Design review of the part shown in the three views and the two pictorial views. Dimensions are in mm from the part's minimum x, y and z. A direction names the side the tool comes from. Give positions to 0.01 mm unless a question says otherwise; leave off trailing zeros. Write each loop counter-clockwise with the first axis right and the second up, starting at its lowest first coordinate (ties: lowest second). Pieces come first, ordered by that corner, then holes. Notation, with made-up numbers: (80, 5.25) -> (94, 5.25) arc R18 cw to (94, 25.25) -> close; hole circle Ø5 at (10.5, 86.25). An arc over 180 degrees is marked (long way). Return JSON: item names as keys, results as strings. Group by question number.
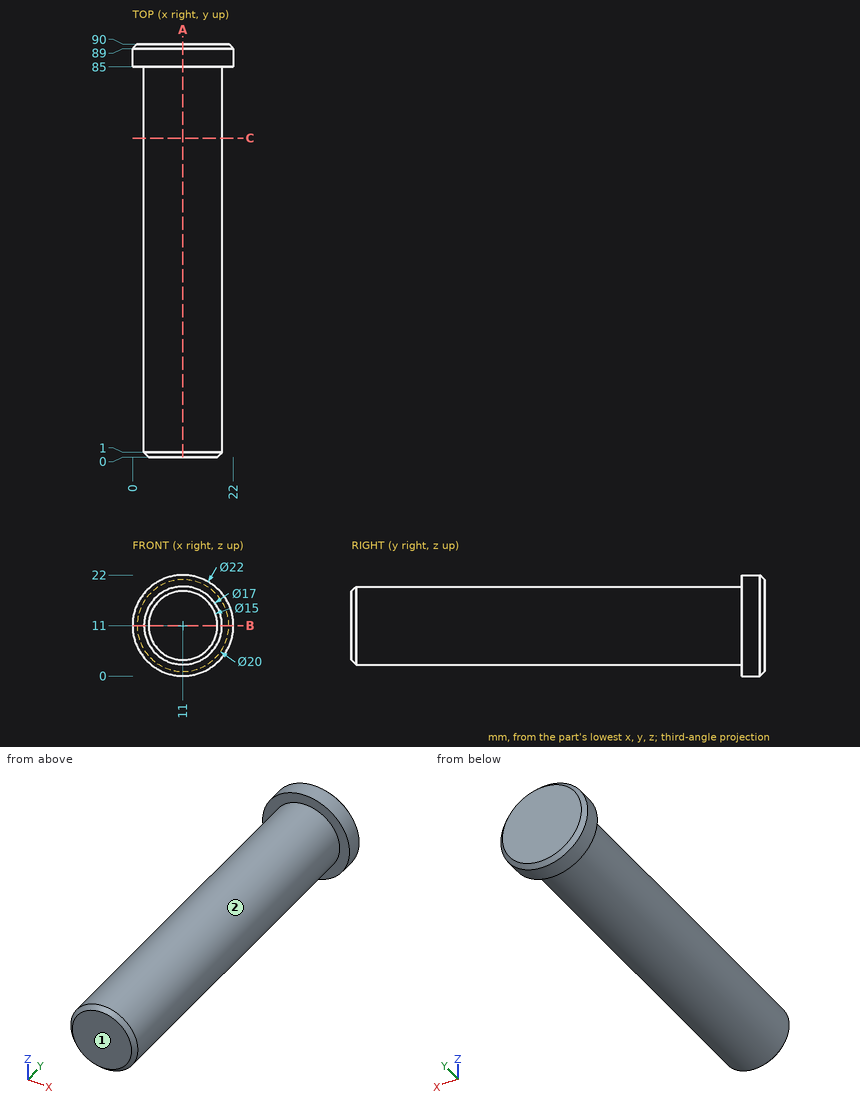
Q1. Take a section at C-C, the plane y = 69.5. Give the boundary of the cut face in (x, z).
Q2. Take a section at A-A, the plane x = 11. Give the boundary of the cut face in (y, z), plus the area to 3 significant figures.
Q3. Tool access review of the marked faces 1 and 2: name each direction out of +Z, -Z, +X, -X, +Y, -Y from which nothing blocks a thin tool from reaching the whole face with its end or side.
Q4. Take a section at B-B, the plane z = 11. Give the boundary of the cut face in (x, y), plus the area to 3 significant figures.
Q5. For L1, parallel to X at y = 71, z = 7; L2, parallel to X at y = 10.5, z = 10.75, list the stretches that pass through material, from the lowest coordinate up. Write a range as from..to.
Q6. Insertion check: pin 1 (10 mm diameter, centred on y = 33.5, z = 16.5, fed in from +X); pin 2 (5 mm diameter, centred on y = 13.5, z = 14.5, fed in from -X); pin 3 (4 mm diameter, centred on x = 9.5, y = 40.5, fed in from +Z). Each pin has a flat end and moves straight along its axis. Give the tip position at first contact, or say it passes through.
Final values:
{
 "1": {"outline": "circle Ø17 at (11, 11)"},
 "2": {"outline": "(0, 3.5) -> (1, 2.5) -> (85, 2.5) -> (85, 0) -> (89, 0) -> (90, 1) -> (90, 21) -> (89, 22) -> (85, 22) -> (85, 19.5) -> (1, 19.5) -> (0, 18.5) -> close", "area": "1,550 mm²"},
 "3": {"face 1": "+Z, -Z, +X, -X, -Y", "face 2": "-Y"},
 "4": {"outline": "(0, 85) -> (2.5, 85) -> (2.5, 1) -> (3.5, 0) -> (18.5, 0) -> (19.5, 1) -> (19.5, 85) -> (22, 85) -> (22, 89) -> (21, 90) -> (1, 90) -> (0, 89) -> close", "area": "1,550 mm²"},
 "5": {"L1": "x = 3.5..18.5", "L2": "x = 2.5..19.5"},
 "6": {"pin 1": "stops at x = 19.49", "pin 2": "stops at x = 2.56", "pin 3": "stops at z = 19.5"}
}
